Geometry: final body of the model. Coordinates: model frame, mm. A direction names the side the tool comes from. Coordinates: 2 decimals unless noted, no trailing zeros. Order: outer loops, then holes, each group sorted by start corner. A loop starts at its lowest first (then second) coordinate and runs counter-clockwise, first axis right, second up. Notation, with made-up numbers: (-28.5, 15) -> (-23.5, 15) arc R27 ccw to (-23.5, 38) -> close; hole circle Ø9 at (-39, 39.5). An arc over 180 degrees is marked (long way). Answer in a Markdown table with one row per item. Add a question column.
1) Section query B-B on x = 0. Return the cut outline in (y, z).
2) Section query A-A on y = 2. Return the cut outline in (x, z), then the cut area to 3 significant figures.
3) Contact query for flat-ended pins moving along their axis: P1, Ø1.5, axis at x = -21.5, y = 2, coming from the -Z side; P2, Ø1, axis at y = 0.5, z = 17.5, coming from the -X side; P3, Ø8, axis at x = -26.5, z = -6.5, coming from the +Y side; P4, Ø12, axis at x = -17.5, z = 14, coming from the -Y side. Output: stop coordinate, or through.
4) Section query D-D on z = 18. Return the cut outline in (x, y).
5) Section query C-C on z = 2. Return the cut outline in (x, y), then the cut area to 3 significant figures.
6) Set-up query: faces 1 (the face through (30.42, 2.46, 9.07)), 2 (the face through (25, 2, 0)), 3 (the face through (0, 5, 10)). Return all of +Z, -Z, +X, -X, +Y, -Y with unobstructed straight access to the full face (end or side cutting, diameter ignored); none if empty.
7) Pull-direction query (Z, two-part tool) for faces 4 (the face through (-25, 2, 0)), 5 (the face through (-30.47, 2.465, 9.084)), 6 (the face through (0, 0, 10)), 7 (the face through (-3, 2, 0)); classes: +Z half, -Z half, draft (parallel to the pull), parting line (faces both ways), or undercut.
8) Ray query, line 1 (Z direction, x = 0, y = 1.1); line 2 (X direction, y = 1.8, z = -2.5); line 3 (Z direction, x = -2.5, y = 0.65). Return the intervals inside material, ascending. Write a range as from..to.
```python
from build123d import *

# Parameters (mm, degrees)
SKETCH1_R           = 3
BOSS_EXTRUDE1_DEPTH = 5


with BuildPart() as part:
    # Sketch1 → Boss-Extrude1 (new body)
    with BuildSketch(Plane(origin=(0, 0, 0), x_dir=(1, 0, 0), z_dir=(0, 1, 0))):
        with BuildLine():
            ThreePointArc((15, 0), (0, 15), (-15, 0))
            Line((-15, 0), (-30, 0))
            Line((-30, 0), (-35, 0))
            Line((-35, 0), (-32.142857143, -9.583148475))
            Line((-32.142857143, -9.583148475), (-28.749445425, -8.571428571))
            ThreePointArc((-28.749445425, -8.571428571), (-23.543039679, -18.593689323), (-15, -25.980762114))
            Line((-15, -25.980762114), (15, -25.980762114))
            ThreePointArc((15, -25.980762114), (23.543039679, -18.593689323), (28.749445425, -8.571428571))
            Line((28.749445425, -8.571428571), (32.142857143, -9.583148475))
            Line((32.142857143, -9.583148475), (35, 0))
            Line((35, 0), (30, 0))
            Line((30, 0), (15, 0))
        make_face()
        Circle(SKETCH1_R, mode=Mode.SUBTRACT)
    extrude(amount=BOSS_EXTRUDE1_DEPTH)


solid = part.part
```
Result:
| question | item | result |
|---|---|---|
| 1 | outline | (0, -15) -> (5, -15) -> (5, -3) -> (0, -3) -> close; (0, 3) -> (5, 3) -> (5, 25.98) -> (0, 25.98) -> close |
| 2 | outline | (-35, 0) -> (-15, 0) arc R15 ccw to (15, 0) -> (35, 0) -> (32.14, 9.58) -> (28.75, 8.57) arc R30 ccw to (15, 25.98) -> (-15, 25.98) arc R30 ccw to (-28.75, 8.57) -> (-32.14, 9.58) -> close; hole circle Ø6 at (0, 0) |
| 2 | area | 1,730 mm2 |
| 3 | P1 | z = 0 |
| 3 | P2 | x = -24.72 |
| 3 | P3 | through |
| 3 | P4 | y = 0 |
| 4 | outline | (-24, 0) -> (24, 0) -> (24, 5) -> (-24, 5) -> close |
| 5 | outline | (-34.4, 0) -> (-2.24, 0) -> (-2.24, 5) -> (-34.4, 5) -> close; (2.24, 0) -> (34.4, 0) -> (34.4, 5) -> (2.24, 5) -> close |
| 5 | area | 322 mm2 |
| 6 | face 1 | +Z, +Y, -Y |
| 6 | face 2 | -Z, +X, +Y, -Y |
| 6 | face 3 | +Z, -Z, +X, -X, +Y |
| 7 | face 4 | -Z half |
| 7 | face 5 | +Z half |
| 7 | face 6 | draft |
| 7 | face 7 | undercut |
| 8 | line 1 | -15..-3, 3..25.98 |
| 8 | line 2 | -14.79..-1.66, 1.66..14.79 |
| 8 | line 3 | -14.79..-1.66, 1.66..25.98 |
